Check sheet for the modelled part. Datum: model origin and axes. Units: mm. A direction names the side the tool comes from. Round coordinates to 2 decimals unless told otherwise and drop trailing zeros. Write each loop counter-clockwise with the first axis right and the second up, starting at its lowest first coordinate (ties: lowest second). Pieces come first, ordered by that corner, then holes. Notation, with made-up numbers: (-24.5, 63.25) -> (-4.5, 63.25) arc R25 ccw to (-4.5, 80.25) -> close; hole circle Ø8 at (78, 59.25). An arc over 180 degrees is marked (long way). One line per item, written item: value.
from build123d import *

# Parameters (mm, degrees)
SKETCH1_W           = 108.2
SKETCH1_H           = 73.5
BOSS_EXTRUDE2_DEPTH = 3.2
SKETCH2_W           = 108.2
SKETCH2_H           = 73.5
SKETCH2_W_2         = 101.8
SKETCH2_H_2         = 67.1
BOSS_EXTRUDE3_DEPTH = 19
SKETCH3_W           = 3.2
SKETCH3_H           = 1
CUT_EXTRUDE1_DEPTH  = 19
SKETCH4_W           = 3.2
SKETCH4_H           = 28.5
CUT_EXTRUDE2_DEPTH  = 19
SKETCH5_W           = 19
SKETCH5_H           = 3.2
SKETCH5_W_2         = 60.7
CUT_EXTRUDE3_DEPTH  = 19
SKETCH6_W           = 3.2
SKETCH6_H           = 16
CUT_EXTRUDE4_DEPTH  = 19
SKETCH7_W           = 9
SKETCH7_H           = 3.2
CUT_EXTRUDE5_DEPTH  = 17
CUT_EXTRUDE6_REACH  = 134.674
SKETCH8_W           = 6
SKETCH8_H           = 8
CUT_EXTRUDE7_REACH  = 134.674
SKETCH9_W           = 6
SKETCH9_H           = 8
SKETCH10_W          = 1.2
SKETCH10_H          = 8
BOSS_EXTRUDE4_DEPTH = 6.5
CUT_EXTRUDE8_REACH  = 139.052
SKETCH11_R          = 2
SKETCH12_W          = 6.5
SKETCH12_H          = 1
BOSS_EXTRUDE5_DEPTH = 10
CHAMFER1_SIZE       = 10
CHAMFER1_SIZE2      = 6.494075932


with BuildPart() as part:
    # Sketch1 → Boss-Extrude2 (new body)
    with BuildSketch(Plane.XY):
        with Locations((54.1, 36.75)):
            Rectangle(SKETCH1_W, SKETCH1_H)
    extrude(amount=BOSS_EXTRUDE2_DEPTH)

    # Sketch2 → Boss-Extrude3 (add)
    with BuildSketch(Plane.XY.offset(3.2)):
        with Locations((54.1, 36.75)):
            Rectangle(SKETCH2_W, SKETCH2_H)
        with Locations((54.1, 36.75)):
            Rectangle(SKETCH2_W_2, SKETCH2_H_2, mode=Mode.SUBTRACT)
    extrude(amount=BOSS_EXTRUDE3_DEPTH)

    # Sketch3 → Cut-Extrude1 (cut)
    with BuildSketch(Plane.XY.offset(22.2)):
        with Locations((1.6, 69.8)):
            Rectangle(SKETCH3_W, SKETCH3_H)
        with Locations((106.6, 69.8)):
            Rectangle(SKETCH3_W, SKETCH3_H)
        with Locations((106.6, 3.7)):
            Rectangle(SKETCH3_W, SKETCH3_H)
        with Locations((1.6, 3.7)):
            Rectangle(SKETCH3_W, SKETCH3_H)
    extrude(amount=-CUT_EXTRUDE1_DEPTH, mode=Mode.SUBTRACT)

    # Sketch4 → Cut-Extrude2 (cut)
    with BuildSketch(Plane.XY.offset(22.2)):
        with Locations((1.6, 34.05)):
            Rectangle(SKETCH4_W, SKETCH4_H)
    extrude(amount=-CUT_EXTRUDE2_DEPTH, mode=Mode.SUBTRACT)

    # Sketch5 → Cut-Extrude3 (cut)
    with BuildSketch(Plane.XY.offset(22.2)):
        with Locations((19.5, 71.9)):
            Rectangle(SKETCH5_W, SKETCH5_H)
        with Locations((67.35, 71.9)):
            Rectangle(SKETCH5_W_2, SKETCH5_H)
    extrude(amount=-CUT_EXTRUDE3_DEPTH, mode=Mode.SUBTRACT)

    # Sketch6 → Cut-Extrude4 (cut)
    with BuildSketch(Plane.XY.offset(22.2)):
        with Locations((106.6, 39.8)):
            Rectangle(SKETCH6_W, SKETCH6_H)
    extrude(amount=-CUT_EXTRUDE4_DEPTH, mode=Mode.SUBTRACT)

    # Sketch7 → Cut-Extrude5 (cut)
    with BuildSketch(Plane.XY.offset(22.2)):
        with Locations((15.5, 1.6)):
            Rectangle(SKETCH7_W, SKETCH7_H)
    extrude(amount=-CUT_EXTRUDE5_DEPTH, mode=Mode.SUBTRACT)

    # Sketch8 → Cut-Extrude6 (cut, up to next)
    with BuildSketch(Plane.ZY, mode=Mode.PRIVATE) as cut_extrude6_sk1:
        with Locations((19.2, 52.3)):
            Rectangle(SKETCH8_W, SKETCH8_H)
    cut_extrude6_tool1 = extrude(cut_extrude6_sk1.sketch, amount=-CUT_EXTRUDE6_REACH, mode=Mode.PRIVATE) & part.part
    add(cut_extrude6_tool1.solids().sort_by_distance((0, 52.3, 19.2))[0], mode=Mode.SUBTRACT)

    # Sketch9 → Cut-Extrude7 (cut, up to next)
    with BuildSketch(Plane(origin=(108.2, 0, 0), x_dir=(0, 0, -1), z_dir=(1, 0, 0)), mode=Mode.PRIVATE) as cut_extrude7_sk1:
        with Locations((-19.2, 20.8)):
            Rectangle(SKETCH9_W, SKETCH9_H)
    cut_extrude7_tool1 = extrude(cut_extrude7_sk1.sketch, amount=-CUT_EXTRUDE7_REACH, mode=Mode.PRIVATE) & part.part
    add(cut_extrude7_tool1.solids().sort_by_distance((108.2, 20.8, 19.2))[0], mode=Mode.SUBTRACT)

    # Sketch10 → Boss-Extrude4 (add)
    with BuildSketch(Plane(origin=(108.2, 0, 0), x_dir=(0, 0, -1), z_dir=(1, 0, 0))):
        with Locations((-15.6, 20.8)):
            Rectangle(SKETCH10_W, SKETCH10_H)
    extrude(amount=BOSS_EXTRUDE4_DEPTH)

    # Sketch11 → Cut-Extrude8 (cut, up to next)
    with BuildSketch(Plane(origin=(0, 0, 15), x_dir=(-1, 0, 0), z_dir=(0, 0, -1)), mode=Mode.PRIVATE) as cut_extrude8_sk1:
        with Locations(Location((-111, 20.8, 0), (0, 0, 90))):
            Circle(SKETCH11_R)
    cut_extrude8_tool1 = extrude(cut_extrude8_sk1.sketch, amount=-CUT_EXTRUDE8_REACH, mode=Mode.PRIVATE) & part.part
    add(cut_extrude8_tool1.solids().sort_by_distance((111, 20.8, 15))[0], mode=Mode.SUBTRACT)

    # Sketch12 → Boss-Extrude5 (add)
    with BuildSketch(Plane(origin=(0, 0, 15), x_dir=(-1, 0, 0), z_dir=(0, 0, -1))):
        with Locations((-111.45, 24.3)):
            Rectangle(SKETCH12_W, SKETCH12_H)
        with Locations((-111.45, 17.3)):
            Rectangle(SKETCH12_W, SKETCH12_H)
    extrude(amount=BOSS_EXTRUDE5_DEPTH)

    # Chamfer1
    chamfer1_edges = [part.edges().sort_by_distance(p)[0] for p in [
        (114.7, 17.3, 5),
        (114.7, 24.3, 5),
    ]]
    chamfer1_side = [part.faces().sort_by_distance(p)[0] for p in [
        (114.7, 20.8, 16.062362796),
    ]]
    chamfer(chamfer1_edges, length=CHAMFER1_SIZE, length2=CHAMFER1_SIZE2, reference=chamfer1_side[0])


solid = part.part
Item 1: Sectioned sample at A-A on x = 111. Enter the section's corners in (y, z).
Answer:
outline: (16.8, 9.3) -> (17.8, 9.3) -> (17.8, 15) -> (18.8, 15) -> (18.8, 16.2) -> (16.8, 16.2) -> close; (22.8, 15) -> (23.8, 15) -> (23.8, 9.3) -> (24.8, 9.3) -> (24.8, 16.2) -> (22.8, 16.2) -> close
Item 2: Depth check by flat-ended pin: P1, Ø7, axis at x = 112.5, z = 12.5, coming from the +Y side; P2, Ø8, axis at y = 25, z = 4, coming from the +X side; P3, Ø1, axis at x = 72, y = 61.5, coming from the +Z side. Enter the tip coordinate at first touch or a pass-through.
Answer:
P1: stops at y = 24.8
P2: stops at x = 110.15
P3: stops at z = 3.2
Item 3: Thickness scan on line 1 (Y direction, x = 100, z = 21.5); line 2 (X direction, y = 51, z = 5.25); line 3 (X direction, y = 20.8, z = 15.55). Record the ranges inside material, lowest first.
Answer:
line 1: y = 0 to 3.2, 70.3 to 73.5
line 2: x = 0 to 3.2, 105 to 108.2
line 3: x = 105 to 109, 113 to 114.7
Item 4: Sectioned sample at D-D on z = 20.5. Count the separate pieces of the cut face and the enclosed holes in it, and give its area (3 significant figures).
Answer:
separate pieces: 10
enclosed holes: 0
area: 632 mm^2
Item 5: Sectioned sample at B-B on y = 54. Enter the section's corners in (x, z).
Answer:
outline: (0, 0) -> (108.2, 0) -> (108.2, 22.2) -> (105, 22.2) -> (105, 3.2) -> (3.2, 3.2) -> (3.2, 16.2) -> (0, 16.2) -> close
Item 6: Tool access check on faces 1 (the flat face through (107, 31.8, 13)), 2 (the flat face through (29, 72, 13)), 3 (the flat face through (2, 48.3, 10)). Record the directions out of +Z, -Z, +X, -X, +Y, -Y that give a thin tool (end or side, any length) a straight path to the whole face; none if there is none.
Answer:
face 1: +Z, +X, -X
face 2: +Z, +Y
face 3: +Z, -X
Item 7: Mould release check, pull along X, two halves, no side actions. Record for faces 4 (the flat face through (108.2, 44, 1)), 5 (the flat face through (37, 72, 13)), 6 (the flat face through (53, 0, 11)): pulls with the +X half, pulls with the -X half, needs draft (parallel to the pull), parting line crosses it, or undercut.
Answer:
face 4: pulls with the +X half
face 5: undercut
face 6: needs draft
Item 8: Sectioned sample at C-C on x = 78.5. Enter the section's corners in (y, z).
Answer:
outline: (0, 0) -> (73.5, 0) -> (73.5, 3.2) -> (3.2, 3.2) -> (3.2, 22.2) -> (0, 22.2) -> close
